```python
from build123d import *

# Parameters (mm, degrees)
SKETCH2_W           = 50
SKETCH2_H           = 50
BOSS_EXTRUDE1_DEPTH = 15.1
SKETCH3_R           = 1.7
CUT_EXTRUDE1_DEPTH  = 73.304979082
SKETCH4_W           = 50
SKETCH4_H           = 12.2
BOSS_EXTRUDE2_DEPTH = 50
SKETCH5_R           = 3
SKETCH5_R_2         = 1.7
CUT_EXTRUDE2_DEPTH  = 91.370625759


with BuildPart() as part:
    # Sketch2 → Boss-Extrude1 (new body)
    with BuildSketch(Plane(origin=(0, 0, 0), x_dir=(0, 1, 0), z_dir=(0, 0, 1))):
        with Locations((25, -25)):
            Rectangle(SKETCH2_W, SKETCH2_H)
    extrude(amount=BOSS_EXTRUDE1_DEPTH)

    # Sketch3 → Cut-Extrude1 (cut, through all)
    with BuildSketch(Plane.XY.offset(15.1)):
        with Locations((16.67, 33.33)):
            Circle(SKETCH3_R)
        with Locations((33.33, 33.33)):
            Circle(SKETCH3_R)
        with Locations((16.67, 16.67)):
            Circle(SKETCH3_R)
        with Locations((33.33, 16.67)):
            Circle(SKETCH3_R)
    extrude(amount=-CUT_EXTRUDE1_DEPTH, mode=Mode.SUBTRACT)

    # Sketch4 → Boss-Extrude2 (add)
    with BuildSketch(Plane.XY.offset(15.1)):
        with Locations((25, 6.1)):
            Rectangle(SKETCH4_W, SKETCH4_H)
    extrude(amount=BOSS_EXTRUDE2_DEPTH)

    # Sketch5 → Cut-Extrude2 (cut, through all)
    with BuildSketch(Plane(origin=(0, 12.2, 0), x_dir=(-1, 0, 0), z_dir=(0, 1, 0))):
        with Locations(Location((-25, 40.1, 0), (0, 0, 90))):
            Circle(SKETCH5_R)
        with Locations(Location((-36, 40.1, 0), (0, 0, 90))):
            Circle(SKETCH5_R_2)
        with Locations(Location((-25, 51.1, 0), (0, 0, 90))):
            Circle(SKETCH5_R_2)
        with Locations(Location((-14, 40.1, 0), (0, 0, 90))):
            Circle(SKETCH5_R_2)
        with Locations(Location((-25, 29.1, 0), (0, 0, 90))):
            Circle(SKETCH5_R_2)
    extrude(amount=-CUT_EXTRUDE2_DEPTH, mode=Mode.SUBTRACT)


solid = part.part
```
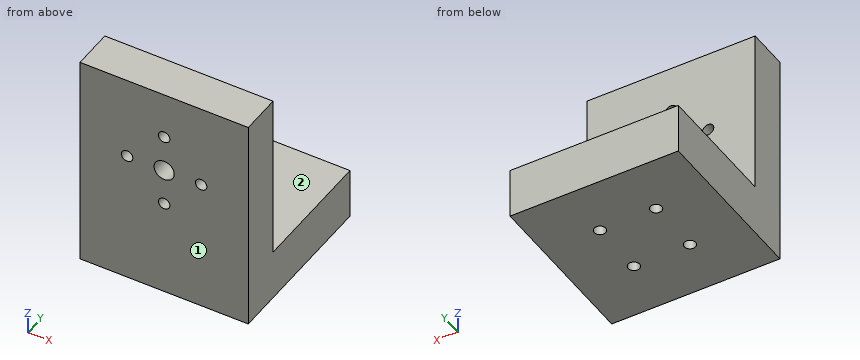
For this review, take the finished solid that the model builds, in its own axes (mm). Face numbers are marked on the shaded views. A direction names the side the tool comes from. Round coordinates to 2 decimals unless told otherwise and drop trailing zeros. Write each loop counter-clockwise with the first axis right and the second up, starting at its lowest first coordinate (ties: lowest second). Pieces come first, ordered by that corner, then holes. Notation, with made-up numbers: (-30.5, -35.5) -> (-25.5, -35.5) arc R8 ccw to (-25.5, -20.5) -> close; hole circle Ø11 at (50, 83). An arc over 180 degrees is marked (long way). One line per question, with ' | ' between items. Start each with the question number.
(1) Tool access review of the marked faces 1 and 2: name each direction out of +Z, -Z, +X, -X, +Y, -Y from which nothing blocks a thin tool from reaching the whole face with its end or side.
(2) Add section D-D, the plane x = 14. Write out the cut boundary in (y, z).
(3) Add section A-A, the plane z = 40.1. Write out the cut boundary in (x, y).
(4) Add section B-B, the plane x = 25. Write out the cut boundary in (y, z).
(5) Add section C-C, the plane z = 29.1. Write out the cut boundary in (x, y).
(6) For line 1 along X through (y, z) = (5, 40); line 2 along Y through (x, z) = (33.33, 4.25); line 3 along X through (y, z) = (5, 51), list the stretches that pass through material, from the lowest coordinate up. Write a range as from..to.
(7) Insertion check: P1, Ø2, axis at x = 25, z = 51.1, coming from the -Y side; P2, Ø5.5, axis at x = 16.67, y = 16.67, coming from the -Z side; P3, Ø5, axis at x = 29, y = 30, coming from the +Z side; P4, Ø6, axis at x = 15, z = 28, coming from the +Y side. Each pin has a flat end and moves straight along its axis. Give the tip position at first contact, or say it passes through.
Answer list:
1) face 1: +Z, -Z, +X, -X, -Y | face 2: +Z, +X, -X, +Y
2) outline: (0, 0) -> (50, 0) -> (50, 15.1) -> (12.2, 15.1) -> (12.2, 38.4) -> (0, 38.4) -> close; (0, 41.8) -> (12.2, 41.8) -> (12.2, 65.1) -> (0, 65.1) -> close
3) outline: (0, 0) -> (12.3, 0) -> (12.3, 12.2) -> (0, 12.2) -> close; (15.7, 0) -> (22, 0) -> (22, 12.2) -> (15.7, 12.2) -> close; (28, 0) -> (34.3, 0) -> (34.3, 12.2) -> (28, 12.2) -> close; (37.7, 0) -> (50, 0) -> (50, 12.2) -> (37.7, 12.2) -> close
4) outline: (0, 0) -> (50, 0) -> (50, 15.1) -> (12.2, 15.1) -> (12.2, 27.4) -> (0, 27.4) -> close; (0, 30.8) -> (12.2, 30.8) -> (12.2, 37.1) -> (0, 37.1) -> close; (0, 43.1) -> (12.2, 43.1) -> (12.2, 49.4) -> (0, 49.4) -> close; (0, 52.8) -> (12.2, 52.8) -> (12.2, 65.1) -> (0, 65.1) -> close
5) outline: (0, 0) -> (23.3, 0) -> (23.3, 12.2) -> (0, 12.2) -> close; (26.7, 0) -> (50, 0) -> (50, 12.2) -> (26.7, 12.2) -> close
6) line 1: 0..12.3, 15.7..22, 28..34.3, 37.7..50 | line 2: 0..14.97, 18.37..31.63, 35.03..50 | line 3: 0..23.3, 26.7..50
7) P1: through | P2: z = 0 | P3: z = 15.1 | P4: y = 12.2
